Autodesk Inventor part; units mm, degrees
ref_plane "YZ Plane" through (0, 0, 0) normal (1, 0, 0) x (0, 1, 0)
ref_plane "XZ Plane" through (0, 0, 0) normal (0, 1, 0) x (-1, 0, 0)
ref_plane "XY Plane" through (0, 0, 0) normal (0, 0, 1) x (1, 0, 0)
sketch "Boceto1" plane through (0, 0, 0) normal (0, 0, 1) x (1, 0, 0)
  circle A0 centre (106.3631, -133) radius 3.5
  line L0 (0, -125) -> (98.3631, -125)
  line L1 (98.3631, -125) -> (98.3631, -85.8745)
  line L2 (0, -140) -> (0, -125)
  line L3 (0, 0) -> (113.3631, 0)
  line L4 (113.3631, 0) -> (113.3631, -60.6726)
  line L5 (0, -15) -> (0, 0)
  circle A1 centre (106.3631, -7) radius 3.5
  arc A2 (98.3631, -54.1255) -> (98.3631, -85.8745) centre (100.3631, -70) ccw
  line L6 (113.3631, -79.3274) -> (113.3631, -140)
  line L7 (113.3631, -140) -> (0, -140)
  line L8 (98.3631, -54.1255) -> (98.3631, -15)
  line L9 (98.3631, -15) -> (0, -15)
  arc A3 (113.3631, -79.3274) -> (113.3631, -60.6726) centre (100.3631, -70) ccw
  circle A4 centre (100.3631, -70) radius 1
  point P0 (98.3631, -85.8745)
  point P1 (113.3631, -79.3274)
  point P2 (113.3631, -60.6726)
  dimension "d0" = 2
extrude "Extrusión1" add sketch "Boceto1" along normal blind 5
properties part number "P7"
Source: CAD feature listing. Evaluate the final solid. Frame: model axes, mm. A direction names the side the tool comes from. Round coordinates to 2 decimals unless told otherwise and drop trailing zeros. Write each loop counter-clockwise with the first axis right and the second up, starting at its lowest first coordinate (ties: lowest second). Pieces come first, ordered by that corner, then holes. Notation, with made-up numbers: M 77.25,69.5 L 91.25,69.5 A12 cw 91.25,76.5 Z; hole C -40,74.25 d2. An arc over 180 degrees is marked long. One line per item, written item: value. Start each with the question number.
Item 1: Mould query, pull axis X, two halves, no side actions, for faces 4 (the cylindrical face through (109.596, -5.659, 2.465)), 5 (the flat face through (98.363, -35, 2)), 6 (the flat face through (113.363, -30, 2)), 7 (the flat face through (50, -15, 2)). Classes: pulls with the +X half, pulls with the -X half, needs draft (parallel to the pull), parting line crosses it, or undercut.
Item 2: Section query C-C (x = 106). Return the cut outline in (y, z).
Item 3: Set-up query: faces 1 (the flat face through (0, -133, 2)), 2 (the flat face through (98.363, -106, 2)), 3 (the flat face through (113.363, -109, 2)). Return all of +Z, -Z, +X, -X, +Y, -Y with unobstructed straight access to the full face (end or side cutting, diameter ignored); none if empty.
Item 4: Pin query (flat end, axial travel): pin 1 (1.5 mm diameter, centred on y = -90.5, z = 3.5, fed in from +X); pin 2 (1.5 mm diameter, centred on y = -36.5, z = 2.5, fed in from -X). Return the tip coordinate at first contact, or that it passes through.
Item 5: Ray query, L1, parallel to X at y = -133, z = 3.65; L2, parallel to Y at x = 26.5, z = 4.55; L3, parallel to X at y = -48.5, z = 4.4. Return the intervals inside material, ascending. Write a range as from..to.
Item 6: Section query B-B (x = 22). Return the cut outline in (y, z), plus the area to 3 significant figures.
Item 7: Section query A-A (y = -133). Return the cut outline in (x, z).
Item 8: Section query D-D (y = -19.5). Return the cut outline in (x, z).
Result set:
1. face 4: undercut
1. face 5: pulls with the -X half
1. face 6: pulls with the +X half
1. face 7: needs draft
2. outline: M -140,0 L -136.48,0 L -136.48,5 L -140,5 Z; M -129.52,0 L -10.48,0 L -10.48,5 L -129.52,5 Z; M -3.52,0 L 0,0 L 0,5 L -3.52,5 Z
3. face 1: +Z, -Z, -X, +Y, -Y
3. face 2: +Z, -Z, -X
3. face 3: +Z, -Z, +X, -Y
4. pin 1: stops at x = 113.36
4. pin 2: stops at x = 98.36
5. L1: x = 0..102.86, 109.86..113.36
5. L2: y = -140..-125, -15..0
5. L3: x = 98.36..113.36
6. outline: M -140,0 L -125,0 L -125,5 L -140,5 Z; M -15,0 L 0,0 L 0,5 L -15,5 Z
6. area: 150 mm²
7. outline: M 0,0 L 102.86,0 L 102.86,5 L 0,5 Z; M 109.86,0 L 113.36,0 L 113.36,5 L 109.86,5 Z
8. outline: M 98.36,0 L 113.36,0 L 113.36,5 L 98.36,5 Z
